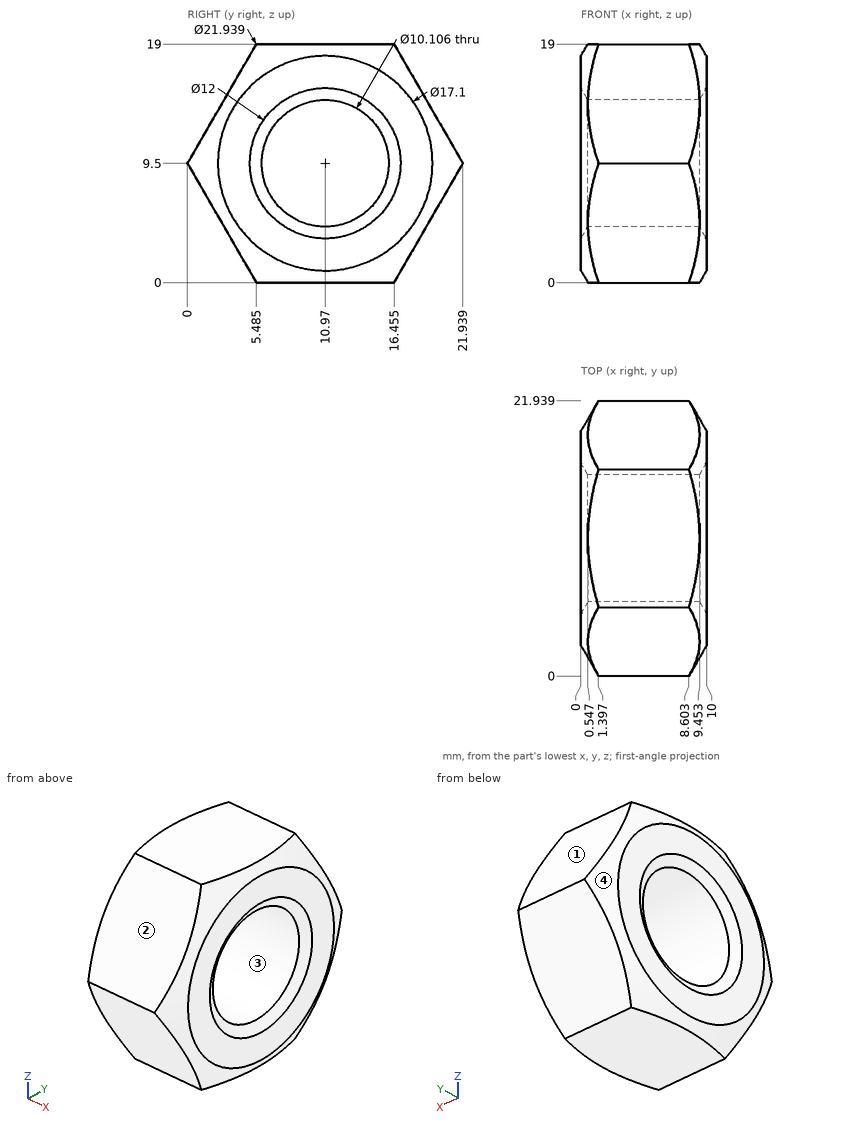
Design review of the part shown in the three views and the two pictorial views. Dimensions are in mm from the part's minimum x, y and z. Coordinates: 2 decimals unless noted, no trailing zeros. One line per question, with ' | ' between items.
(1) Wall thickness on probe 1 along Y at (x, z) = (6, 6.75); probe 2 along Z at (x, y) = (8.5, 8); probe 3 along Y at (x, z) = (3, 6) (1 decimal): over which ranges is each line inside the solid? List them lowest first.
Filled in:
probe 1: y = 1.59 to 6.73, 15.21 to 20.35 | probe 2: z = 0 to 5.41, 13.59 to 19 | probe 3: y = 2 to 7.3, 14.6 to 19.9
(2) Draft analysis for pull direction Y (two halves, no side actions). For the marked faces 1, 2, 3 and 4, state which applies: released by +Y, released by -Y, zero draft, split by the parting line, or undercut.
Filled in:
face 1: released by +Y | face 2: released by -Y | face 3: undercut | face 4: split by the parting line
(3) For pin 1 Ø1.5 at (y, z) = (14.5, 10) entering from +X; pin 2 Ø5 at (x, z) = (3, 4) entering from +Y; pin 3 Ø2 at (y, z) = (11.5, 14) entering from +X; pin 4 Ø2 at (x, y) = (1.5, 19) entering from +Z (1 decimal), all flat-tipped, find the tip position at first contact; note any pin that passes through.
Filled in:
pin 1: passes through | pin 2: stops at y = 20.21 | pin 3: stops at x = 9.73 | pin 4: stops at z = 16.3
